Could you check a few things on this model? Use its own coordinates, in mm. Face numbers are marked on the shaded views. A direction names the side the tool comes from. Give positions to 0.01 mm unless a question says otherwise; leave off trailing zeros. Write each loop counter-clockwise with the first axis right and the second up, starting at its lowest first coordinate (ties: lowest second). Pieces come first, ordered by that corner, then holes. Notation, with made-up numbers: M 49.5,36 L 67.5,36 A21 cw 67.5,70 Z; hole C -40,59 d9. An arc over 180 degrees is marked long. Answer as a JSON object with one key per item and string values. Group by question number.
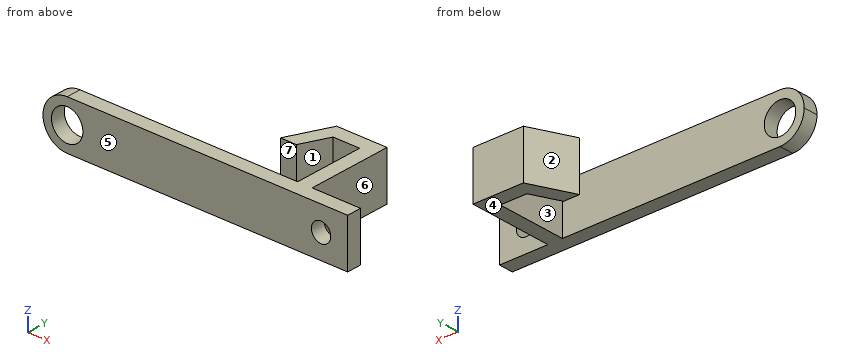
```python
from build123d import *

# Parameters (mm, degrees)
F0_W     = 50
F0_H     = 3
F1_DEPTH = 10
F3_D     = 4
F5_R     = 4.99999
F6_D     = 6.5


# Not quite as in the source:
# - a fillet or chamfer is up to 0.001 mm smaller than in the source, because OpenCascade refuses the exact size


with BuildPart() as f1:
    # F0 (on Top) → F1 (new body)
    with BuildSketch(Plane.XY):
        Polygon((-2.2981421612, -11.8900760232), (10.7018578388, -11.8900760232), (10.7018578388, -8.8900760232), (0.7018578388, -8.8900760232), (0.7018578388, 8.6099239768), (-9.7093529436, 8.6099239768), (-13.7242264302, 0), (-10.4140926733, 0), (-7.7981421612, 5.6099239768), (-2.2981421612, 5.6099239768), (-2.2981421612, -8.8900760232), align=None)
        with Locations((-27.2981421612, -10.3900760232)):
            Rectangle(F0_W, F0_H)
    extrude(amount=F1_DEPTH)

    # F3 (through all)
    with Locations(Plane(origin=(0, -8.8900760232, 0), x_dir=(-1, 0, 0), z_dir=(0, 1, 0))):
        with Locations((-5.2018578388, 5)):
            Hole(F3_D / 2)

    # F5 (radius 5 in the source; OpenCascade refuses exactly that, so slightly less here)
    f5_edges = [f1.edges().sort_by_distance(p)[0] for p in [
        (-52.298142, -10.390076, 10),
        (-52.298142, -10.390076, 0),
    ]]
    fillet(f5_edges, radius=F5_R)

    # F6 (through all)
    with Locations(Plane.XZ.offset(11.8900760232)):
        with Locations((-47.2981421612, 5)):
            Hole(F6_D / 2)


solid = f1.part
```
1) For the marked faces 5, 6 and 7, which set-ups out of +Z, -Z, +X, -X, +Y, -Y let a thin tool reach every point of the face, with its end or its side?
2) Please list where these lines run through material, in increasing order: line 1 along Y through (x, z) = (1, 3.75); line 2 along Y through (x, z) = (-7, 7.5); line 3 along X through (y, z) = (-5.75, 2.5). Write a range as from..to.
3) If we section it at C-C, the plane z = 5.75: List the corners of the cut face in (x, y) for me.
4) I'm going to push flat-ended pins straight in: pin 1 (5 mm diameter, centred on x = -17.5, z = 1.5, fed in from +Y); pin 2 (5 mm diameter, centred on y = -1.5, z = 5, fed in from +X). Where does each tip first touch, or does it pass through?
5) We'd pull the mould along X, two halves only. Please class the marked faces 1, 2, 3 and 4: released by +X, released by -X, zero draft, split by the parting line, or undercut.
6) If we section it at D-D, the plane y = 6.75: List the corners of the cut face in (x, z) for me.
7) If we section it at A-A, the plane x = 6: List the corners of the cut face in (y, z) for me.
8) If we section it at B-B, the plane y = 4.25: List the corners of the cut face in (x, z) for me, plus the area to 3 significant figures.
Taken from the geometry:
{
 "1": {"face 5": "+Z, -Z, +X, -X, -Y", "face 6": "+Z, -Z, +X, +Y", "face 7": "+Z, -Z, -X"},
 "2": {"line 1": "-11.89..-8.89", "line 2": "-11.89..-8.89, 5.61..8.61", "line 3": "-2.3..0.7"},
 "3": {"outline": "M -52.24,-11.89 L -50.46,-11.89 L -50.46,-8.89 L -52.24,-8.89 Z; M -44.14,-11.89 L 3.35,-11.89 L 3.35,-8.89 L 0.7,-8.89 L 0.7,8.61 L -9.71,8.61 L -13.72,0 L -10.41,0 L -7.8,5.61 L -2.3,5.61 L -2.3,-8.89 L -44.14,-8.89 Z; M 7.06,-11.89 L 10.7,-11.89 L 10.7,-8.89 L 7.06,-8.89 Z"},
 "4": {"pin 1": "y = -8.89", "pin 2": "x = 0.7"},
 "5": {"face 1": "undercut", "face 2": "released by -X", "face 3": "undercut", "face 4": "zero draft"},
 "6": {"outline": "M -10.58,0 L 0.7,0 L 0.7,10 L -10.58,10 Z"},
 "7": {"outline": "M -11.89,0 L -8.89,0 L -8.89,3.17 L -11.89,3.17 Z; M -11.89,6.83 L -8.89,6.83 L -8.89,10 L -11.89,10 Z"},
 "8": {"outline": "M -11.74,0 L -8.43,0 L -8.43,10 L -11.74,10 Z; M -2.3,0 L 0.7,0 L 0.7,10 L -2.3,10 Z", "area": "63.1 mm²"}
}
